from build123d import *

# Parameters (mm, degrees)
F2_R     = 17.1
F3_DEPTH = 12
F6_W     = 15.8
F6_H     = 20
F7_DEPTH = 13.5


with BuildPart() as f1:
    # F0 (on Front) → F1 (revolve)
    with BuildSketch(Plane.XZ):
        with BuildLine():
            Line((27.9, 20), (322.9, 20))
            Line((322.9, 20), (322.9, 22.5))
            Line((322.9, 22.5), (199.2, 22.5))
            ThreePointArc((199.2, 22.5), (197.9, 21.2), (196.6, 22.5))
            Line((196.6, 22.5), (27.9, 22.5))
            Line((27.9, 22.5), (27.9, 20))
        make_face()
        with BuildLine():
            ThreePointArc((25.4, 0), (26.027422517, 10.0778221854), (27.9, 20))
            Line((27.9, 20), (27.9, 22.5))
            ThreePointArc((27.9, 22.5), (24.1650624277, 11.5244305716), (22.9, 0))
            Line((22.9, 0), (25.4, 0))
        make_face()
    revolve(axis=Axis((175.4, 0, 0), (1, 0, 0)))

    # F2 (on Front) → F3 (join, symmetric)
    with BuildSketch(Plane.XZ):
        with BuildLine():
            ThreePointArc((16.1248255805, -12), (19.0803432119, -6.320641021), (20.1, 0))
            ThreePointArc((20.1, 0), (19.0803432119, 6.320641021), (16.1248255805, 12))
            ThreePointArc((16.1248255805, 12), (-20.1, 0), (16.1248255805, -12))
        make_face()
        Circle(F2_R, mode=Mode.SUBTRACT)
        with BuildLine():
            ThreePointArc((16.1248255805, 12), (19.0803432119, 6.320641021), (20.1, 0))
            ThreePointArc((20.1, 0), (19.0803432119, -6.320641021), (16.1248255805, -12))
            Line((16.1248255805, -12), (26.1248255805, -12))
            Line((26.1248255805, -12), (26.1248255805, 12))
            Line((26.1248255805, 12), (16.1248255805, 12))
        make_face()
    extrude(amount=F3_DEPTH, both=True)



with BuildPart() as f5:
    # F4 (on Front) → F5 (revolve)
    with BuildSketch(Plane.XZ):
        Polygon((33.445, 78), (166.9, 78), (166.9, 80.5), (30.9, 80.5), (30.9, 58), (33.445, 58), align=None)
    revolve(axis=Axis((98.9, 0, 58), (1, 0, 0)))


with BuildPart() as f1_1:
    add(f1.part)

    add(f5.part)  # F7 merges F5
    # F6 (on Front) → F7 (join, symmetric)
    with BuildSketch(Plane.XZ):
        with Locations((42, 29)):
            Rectangle(F6_W, F6_H)
    extrude(amount=F7_DEPTH, both=True)


solid = f1_1.part
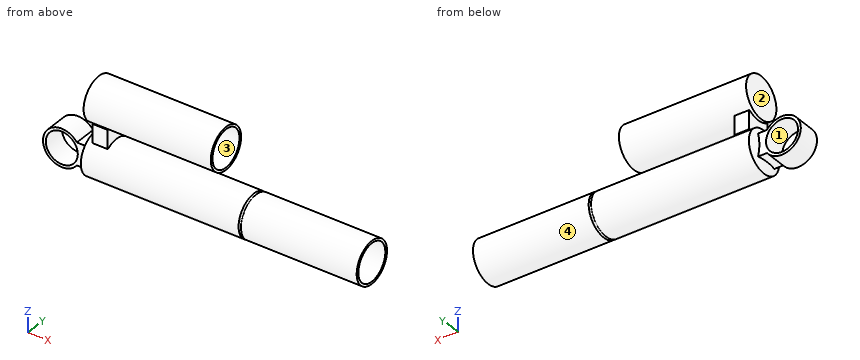
Verification items for the finished model (mm, model axes). Face numbers are marked on the shaded views. Round coordinates to 2 decimals unless told otherwise and drop trailing zeros. Loops run counter-clockwise (first coordinate to the right, second up) from the corner with the lowest first, then second, coordinate; pieces in that order, holes last. Notation, with made-up numbers: (-12, 22) - (43, 22) arc R19 ccw to (43, 34) - close; hole circle Ø1 at (47.5, 33.5). An arc over 180 degrees is marked (long way). Answer in a Markdown table with one row per item. Add a question column.
Q1. Gauge pin test, flat ends, axial feed: pin 1 (10 mm diameter, centred on y = -6.5, z = 32.5, fed in from -X); pin 2 (0.7 mm diameter, centred on x = 44, y = 12.5, fed in from -Z); pin 3 (4 mm diameter, centred on y = 15, z = 68.5, fed in from +X); pin 4 (20 mm diameter, centred on x = -5, z = 3, fed in from +Y). Record the tip position at first contact, or that the pin passes through.
Q2. Material ranges on line 1 (Z direction, x = 126, y = 0); line 2 (Y direction, x = 255, z = 0); line 3 (Z direction, x = 34, y = 3.5), recorded low to high.
Q3. Release check for a two-part mould opening along Z. For the marked faces 1, 2, 3 and 4 record: pulls with the +Z half, pulls with the -Z half, needs draft (parallel to the pull), parting line crosses it, or undercut.
Q4. Section check D-D on x = 268. Enter the section's corners in (y, z), plus the area to 3 significant figures.
Q5. Section check C-C on x = 105. Enter the section's corners in (y, z).
Q6. Section check A-A on z = 0. Enter the section's corners in (x, y) (3 decimals).
Q7. Section check B-B on x = 0. Enter the section's corners in (y, z).
Found:
| question | item | result |
|---|---|---|
| 1 | pin 1 | stops at x = 30.9 |
| 1 | pin 2 | stops at z = -18.94 |
| 1 | pin 3 | stops at x = 166.9 |
| 1 | pin 4 | passes through |
| 2 | line 1 | z = -22.5 to -20, 20 to 22.5, 35.5 to 38, 78 to 80.5 |
| 2 | line 2 | y = -22.5 to -20, 20 to 22.5 |
| 2 | line 3 | z = -22.23 to -19.69, 19.69 to 22.23, 35.77 to 38.31, 77.69 to 80.23 |
| 3 | face 1 | undercut |
| 3 | face 2 | needs draft |
| 3 | face 3 | undercut |
| 3 | face 4 | parting line crosses it |
| 4 | outline | circle Ø45 at (0, 0); hole circle Ø40 at (0, 0) |
| 4 | area | 334 mm² |
| 5 | outline | circle Ø45 at (0, 0); circle Ø45 at (0, 58); hole circle Ø40 at (0, 0); hole circle Ø40 at (0, 58) |
| 6 | outline | (-20.1, -12) - (-17.1, -12) - (-17.1, 12) - (-20.1, 12) - close; (17.1, -12) - (24.273, -12) arc R53.125 ccw to (27.9, -22.5) - (196.6, -22.5) arc R1.3 cw to (199.2, -22.5) - (322.9, -22.5) - (322.9, -20) - (27.9, -20) arc R81.25 cw to (26.125, -10.829) - (26.125, 10.829) arc R81.25 cw to (27.9, 20) - (322.9, 20) - (322.9, 22.5) - (199.2, 22.5) arc R1.3 cw to (196.6, 22.5) - (27.9, 22.5) arc R53.125 ccw to (24.273, 12) - (17.1, 12) - close |
| 7 | outline | (-12, -20.1) - (12, -20.1) - (12, -17.1) - (-12, -17.1) - close; (-12, 17.1) - (12, 17.1) - (12, 20.1) - (-12, 20.1) - close |
